Part model, mm, in its own coordinate system. Round coordinates to 2 decimals unless told otherwise and drop trailing zeros. Loops run counter-clockwise (first coordinate to the right, second up) from the corner with the lowest first, then second, coordinate; pieces in that order, holes last.
from build123d import *

# Parameters (mm, degrees)
F0_W     = 16
F0_H     = 11
F1_DEPTH = 26
F6_DEPTH = 19.82577


with BuildPart() as f1:
    # F0 (on Front) → F1 (new body)
    with BuildSketch(Plane.XZ):
        Rectangle(F0_W, F0_H)
    extrude(amount=-F1_DEPTH)

    # F4 (on offset) → F5 (revolve, cut)
    with BuildSketch(Plane(origin=(-1.6, 0, 0), x_dir=(0, -1, 0), z_dir=(-1, 0, 0))):
        Polygon((-26, -0.7), (0, -0.7), (0, 3.1), (-26, 0.8), align=None)
    revolve(axis=Axis((-1.6, 13, -0.7), (0, 1, 0)), mode=Mode.SUBTRACT)

    # F2 (on face) → F6 (cut)
    with BuildSketch(Plane(origin=(-8, 0, 0), x_dir=(0, -1, 0), z_dir=(-1, 0, 0))):
        Polygon((-26, 5.5), (-26, 1.1), (0, 5.5), align=None)
    extrude(amount=-F6_DEPTH, mode=Mode.SUBTRACT)


solid = f1.part
1) Mould opens along Z. For faces 1 (the face through (8, 13, -1)), 2 (the face through (-0.11, 13.18, 3.27)), 3 (the face through (-0.809, 13.182, 1.812)) say: released by +Z, released by -Z, zero draft, split by the parting line, or undercut.
Values:
face 1: zero draft
face 2: released by +Z
face 3: undercut
2) Slice it at C-C, the plane y = 16.5. Give the cut face in (x, z).
Values:
outline: (-8, -5.5) - (8, -5.5) - (8, 2.71) - (-8, 2.71) - close; hole circle Ø4.68 at (-1.6, -0.7)
3) Drop flat-ended pins along their axis: pin 1 Ø4 at (x, z) = (-2, 4) entering from -Y; pin 2 Ø5 at (x, y) = (-2, 21) entering from +Z. Give the stop position or say it passes through.
Values:
pin 1: stops at y = 0
pin 2: stops at z = 2.37
4) Slice it at B-B, the plane x = -1.6. Give the cut face in (y, z).
Values:
outline: (0, -5.5) - (26, -5.5) - (26, -2.2) - (0, -4.5) - close; (0, 3.1) - (26, 0.8) - (26, 1.1) - (0, 5.5) - close
5) Slice it at D-D, the plane x = 4.75. Give the cut face in (y, z), then the cut area to 3 significant figures.
Values:
outline: (0, -5.5) - (26, -5.5) - (26, 1.1) - (0, 5.5) - close
area: 229 mm2
6) Wall check: line 1 along X through (y, z) = (13.5, -2.25); line 2 along Z through (x, y) = (-2.5, 20.75); line 3 along X through (y, z) = (2.5, 2). Give the ranges that are in metal, low to high.
Values:
line 1: x = -8 to -3.69, 0.49 to 8
line 2: z = -5.5 to -2.45, 1.05 to 1.99
line 3: x = -8 to -3.95, 0.75 to 8
7) Slice it at A-A, the plane z = -0.7. Give the cut face in (x, y), then the cut area to 3 significant figures.
Values:
outline: (-8, 0) - (-5.4, 0) - (-3.1, 26) - (-8, 26) - close; (-0.1, 26) - (2.2, 0) - (8, 0) - (8, 26) - close
area: 278 mm2
